Check sheet for the modelled part. Datum: model origin and axes. Units: mm. A direction names the side the tool comes from. Give positions to 0.01 mm unless a question says otherwise; leave off trailing zeros. Order: outer loops, then holes, each group sorted by start corner. A loop starts at its lowest first (then second) coordinate and runs counter-clockwise, first axis right, second up. Notation, with made-up numbers: (78.25, -8.75) -> (108.25, -8.75) arc R15 ccw to (108.25, -4.75) -> close; hole circle Ø2 at (15, -1). An arc over 180 degrees is marked (long way). One line per question, with ' | ' between items.
```python
from build123d import *

# Parameters (mm, degrees)
F1_DEPTH = 30
F2_DEPTH = 22


with BuildPart() as f1:
    # F0 (on Front) → F1 (new body)
    with BuildSketch(Plane.XZ):
        Polygon((0, 15), (-12.990381, 7.5), (-12.990381, -7.5), (0, -15), (12.990381, -7.5), (12.990381, 7.5), align=None)
        with BuildLine():
            ThreePointArc((-9.5, 0), (0, 9.5), (9.5, 0))
            ThreePointArc((9.5, 0), (0, -9.5), (-9.5, 0))
        make_face(mode=Mode.SUBTRACT)
        with BuildLine():
            ThreePointArc((-9.5, 0), (0, -9.5), (9.5, 0))
            ThreePointArc((9.5, 0), (0, 9.5), (-9.5, 0))
        make_face()
        with BuildLine():
            ThreePointArc((1.5, 0), (-3.5, -5), (-8.5, 0))
            ThreePointArc((-8.5, 0), (-3.5, 5), (1.5, 0))
        make_face(mode=Mode.SUBTRACT)
    extrude(amount=F1_DEPTH)


with BuildPart() as f2:
    # F0 (on Front) → F2 (new body)
    with BuildSketch(Plane.XZ):
        with BuildLine():
            ThreePointArc((-9.5, 0), (0, -9.5), (9.5, 0))
            ThreePointArc((9.5, 0), (0, 9.5), (-9.5, 0))
        make_face()
        with BuildLine():
            ThreePointArc((1.5, 0), (-3.5, -5), (-8.5, 0))
            ThreePointArc((-8.5, 0), (-3.5, 5), (1.5, 0))
        make_face(mode=Mode.SUBTRACT)
        with BuildLine():
            ThreePointArc((1.5, 0), (-3.5, 5), (-8.5, 0))
            ThreePointArc((-8.5, 0), (-3.5, -5), (1.5, 0))
        make_face()
    extrude(amount=F2_DEPTH)


with BuildPart() as f1_1:
    add(f1.part)

    # F3: cut F2
    add(f2.part, mode=Mode.SUBTRACT)


solid = f1_1.part
```
Q1. Section check C-C (x = -3.5). Enter the section's corners in (y, z).
Result sheet:
outline: (-30, -12.98) -> (0, -12.98) -> (0, -8.83) -> (-22, -8.83) -> (-22, -5) -> (-30, -5) -> close; (-30, 5) -> (-22, 5) -> (-22, 8.83) -> (0, 8.83) -> (0, 12.98) -> (-30, 12.98) -> close
Q2. Mould release check, pull along Z, two halves, no side actions. Record for faces 1 (the face through (3, -30, 0)), 2 (the face through (2, -22, 0)), 3 (the face through (-6.404, -14.79, 11.302)), 4 (the face through (-6.586, -14.79, -11.198)): pulls with the +Z half, pulls with the -Z half, needs draft (parallel to the pull), parting line crosses it, or undercut.
Result sheet:
face 1: needs draft | face 2: undercut | face 3: pulls with the +Z half | face 4: pulls with the -Z half
Q3. Thickness scan on line 1 (Z direction, x = 0, y = -8); line 2 (Y direction, x = -2.75, z = -6.5); line 3 (X direction, y = -19.5, z = 2.5). Record the ranges inside material, lowest first.
Result sheet:
line 1: z = -15 to -9.5, 9.5 to 15 | line 2: y = -30 to -22 | line 3: x = -12.99 to -9.17, 9.17 to 12.99
Q4. Section check A-A (z = 0). Enter the section's corners in (x, y).
Result sheet:
outline: (-12.99, -30) -> (-8.5, -30) -> (-8.5, -22) -> (-9.5, -22) -> (-9.5, 0) -> (-12.99, 0) -> close; (1.5, -30) -> (12.99, -30) -> (12.99, 0) -> (9.5, 0) -> (9.5, -22) -> (1.5, -22) -> close
Q5. Access from +Z, -Z, +X, -X, +Y, -Y to the whole of each face (thin tool, end or side, straight path). Record for faces 5 (the face through (-2.059, -10.846, -9.274)), 6 (the face through (-12.99, -15, 0)).
Result sheet:
face 5: +Y | face 6: +Z, -Z, -X, +Y, -Y
Q6. Section check B-B (y = -24). Enter the section's corners in (x, z).
Result sheet:
outline: (-12.99, -7.5) -> (0, -15) -> (12.99, -7.5) -> (12.99, 7.5) -> (0, 15) -> (-12.99, 7.5) -> close; hole circle Ø10 at (-3.5, 0)
Q7. Section check D-D (z = -6.75). Enter the section's corners in (x, y).
Result sheet:
outline: (-12.99, -30) -> (12.99, -30) -> (12.99, 0) -> (6.68, 0) -> (6.68, -22) -> (-6.68, -22) -> (-6.68, 0) -> (-12.99, 0) -> close
Q8. Depth check by flat-ended pin: pin 1 Ø5 at (x, y) = (9.5, -24.5) entering from +Z; pin 2 Ø5 at (x, y) = (6.5, -9) entering from -Z; pin 3 Ø8 at (x, z) = (-3.5, 0) entering from -Y; pin 4 Ø1.5 at (x, y) = (-1, -13) entering from +Z. Enter the tip coordinate at first touch or a pass-through.
Result sheet:
pin 1: stops at z = 10.96 | pin 2: stops at z = -12.69 | pin 3: passes through | pin 4: stops at z = 14.86
